Build history of the part. All positions in model axes, mm. Face numbers are marked on the shaded views. A direction names the side the tool comes from. Give positions to 0.01 mm unless a question says otherwise; leave off trailing zeros. Write each loop counter-clockwise with the first axis right and the second up, starting at its lowest first coordinate (ties: lowest second). Pieces come first, ordered by that corner, then holes. Notation, with made-up numbers: (88, 48.25) -> (125, 48.25) arc R17 cw to (125, 77.25) -> close; hole circle Ø4 at (84, 74). An arc over 180 degrees is marked (long way). Write item = value, one per line. Start each with the question number.
Q1. Tool access for the marked faces 1 and 2: list every direction of +Z, -Z, +X, -X, +Y, -Y with a clear straight run to the whole face (end or side of a thin tool).
Q2. Saw through at B-B, the plane z = 58. List the corners of the cut face in (x, y), then the cut area to 3 significant figures.
Q3. Saw through at D-D, the plane z = 139. List the corners of the cut face in (x, y).
Q4. Wall check: line 1 (Y direction, x = 21, z = -143); line 2 (X direction, y = 10.5, z = -98.5); line 3 (Y direction, x = -23, z = -87.5). Give the ranges that are in metal, low to high.
Q5. Drop flat-ended pins along their axis: P1, Ø6, axis at y = 5, z = 59.5, coming from the +X side; P2, Ø1.7, axis at y = 4.5, z = -142, coming from the -X side; P3, Ø12, axis at x = -7, z = -20, coming from the +Y side; P4, Ø6, axis at x = 12, z = -29.5, coming from the -Y side. Give the stop position or say it passes through.
Q6. Saw through at C-C, the plane z = -123. List the corners of the cut face in (x, y).
Q7. Saw through at A-A, the plane z = -68. List the corners of the cut face in (x, y), then the cut area to 3 significant figures.
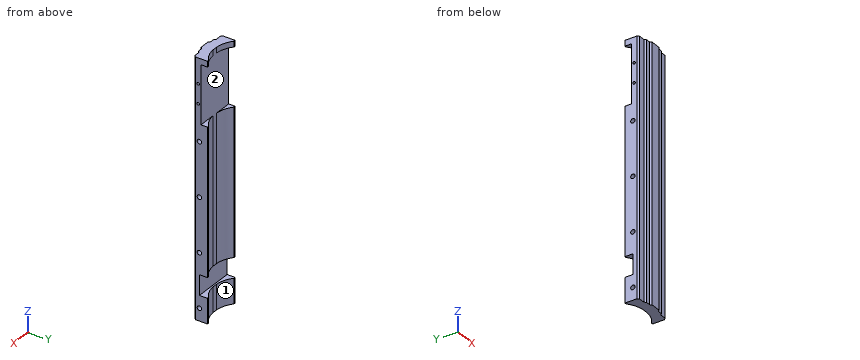
from build123d import *

# Parameters (mm, degrees)
SKETCH1_W               = 50
SKETCH1_H               = 317
BOSS_EXTRUDE1_DEPTH     = 7
BOSS_EXTRUDE2_DEPTH     = 317
SKETCH4_W               = 50
SKETCH4_H               = 72.5
CUT_EXTRUDE2_DEPTH      = 15
CUT_EXTRUDE3_DEPTH      = 12.5
CUT_EXTRUDE3_DEPTH_BACK = 2
SKETCH5_W               = 50
SKETCH5_H               = 25
SKETCH6_R               = 1.6
CUT_EXTRUDE4_DEPTH      = 4.5
SKETCH7_R               = 2.8
CUT_EXTRUDE5_DEPTH      = 9.1
LPATTERN2_COUNT         = 4
LPATTERN2_PITCH         = 67
MIRROR3_COPY_1_SKETCH_R = 2.8
MIRROR3_COPY_1_DEPTH    = 9.1
MIRROR3_COPY_2_SKETCH_R = 2.8
MIRROR3_COPY_2_DEPTH    = 9.1
MIRROR3_COPY_3_SKETCH_R = 2.8
MIRROR3_COPY_3_DEPTH    = 9.1
BOSS_EXTRUDE3_DEPTH     = 317


with BuildPart() as part:
    # Sketch1 → Boss-Extrude1 (new body)
    with BuildSketch(Plane(origin=(0, 0, 0), x_dir=(1, 0, 0), z_dir=(0, 1, 0))):
        Rectangle(SKETCH1_W, SKETCH1_H)
    extrude(amount=BOSS_EXTRUDE1_DEPTH)

    # Sketch2 → Boss-Extrude2 (add)
    with BuildSketch(Plane.XY.offset(158.5)):
        with BuildLine():
            Line((25, 0), (25, 15))
            Line((25, 15), (23, 15))
            ThreePointArc((23, 15), (12.243394569, 8.789970948), (-0.047456713, 7))
            Line((-0.047456713, 7), (-0.047456713, 0))
            Line((-0.047456713, 0), (25, 0))
        make_face()
    boss_extrude2 = extrude(amount=-BOSS_EXTRUDE2_DEPTH)

    # Mirror1: Boss-Extrude2 across plane
    add(boss_extrude2.mirror(Plane(origin=(0, 0, 0), x_dir=(0, 0, 1), z_dir=(1, 0, 0))))

    # Sketch4 → Cut-Extrude2 (cut)
    with BuildSketch(Plane(origin=(0, 7, 0), x_dir=(1, 0, 0), z_dir=(0, 1, 0))):
        with Locations((0, -115.25)):
            Rectangle(SKETCH4_W, SKETCH4_H)
    extrude(amount=CUT_EXTRUDE2_DEPTH, mode=Mode.SUBTRACT)

    # Sketch5 → Cut-Extrude3 (cut, two sides: drawn at the far end of the back side and taken through both)
    with BuildSketch(Plane(origin=(0, 7, 0), x_dir=(1, 0, 0), z_dir=(0, 1, 0)).offset(-CUT_EXTRUDE3_DEPTH_BACK)):
        with Locations((0, 115)):
            Rectangle(SKETCH5_W, SKETCH5_H)
    extrude(amount=CUT_EXTRUDE3_DEPTH + CUT_EXTRUDE3_DEPTH_BACK, mode=Mode.SUBTRACT)

    # Sketch6 → Cut-Extrude4 (cut)
    with BuildSketch(Plane.ZY.offset(25)):
        with Locations((103.166666667, 3.5)):
            Circle(SKETCH6_R)
        with Locations((127.333333333, 3.5)):
            Circle(SKETCH6_R)
    cut_extrude4 = extrude(amount=-CUT_EXTRUDE4_DEPTH, mode=Mode.SUBTRACT)

    # Sketch7 → Cut-Extrude5 (cut)
    with BuildSketch(Plane(origin=(25, 0, 0), x_dir=(0, 0, -1), z_dir=(1, 0, 0))):
        with Locations((143, 5)):
            Circle(SKETCH7_R)
    cut_extrude5 = extrude(amount=-CUT_EXTRUDE5_DEPTH, mode=Mode.SUBTRACT)

    # LPattern2: Cut-Extrude5 ×4
    with Locations(*[(0, 0, i * LPATTERN2_PITCH) for i in range(1, LPATTERN2_COUNT)]):
        add(cut_extrude5, mode=Mode.SUBTRACT)

    # Mirror3: Cut-Extrude4, Cut-Extrude5 across plane
    add(cut_extrude4.mirror(Plane(origin=(0, 0, 0), x_dir=(0, 0, 1), z_dir=(1, 0, 0))), mode=Mode.SUBTRACT)
    add(cut_extrude5.mirror(Plane(origin=(0, 0, 0), x_dir=(0, 0, 1), z_dir=(1, 0, 0))), mode=Mode.SUBTRACT)

    # Mirror3 copy 1 sketch → Mirror3 copy 1 (cut)
    with BuildSketch(Plane(origin=(-25, 0, 67), x_dir=(0, 0, -1), z_dir=(-1, 0, 0))):
        with Locations((143, -5)):
            Circle(MIRROR3_COPY_1_SKETCH_R)
    extrude(amount=-MIRROR3_COPY_1_DEPTH, mode=Mode.SUBTRACT)

    # Mirror3 copy 2 sketch → Mirror3 copy 2 (cut)
    with BuildSketch(Plane(origin=(-25, 0, 134), x_dir=(0, 0, -1), z_dir=(-1, 0, 0))):
        with Locations((143, -5)):
            Circle(MIRROR3_COPY_2_SKETCH_R)
    extrude(amount=-MIRROR3_COPY_2_DEPTH, mode=Mode.SUBTRACT)

    # Mirror3 copy 3 sketch → Mirror3 copy 3 (cut)
    with BuildSketch(Plane(origin=(-25, 0, 201), x_dir=(0, 0, -1), z_dir=(-1, 0, 0))):
        with Locations((143, -5)):
            Circle(MIRROR3_COPY_3_SKETCH_R)
    extrude(amount=-MIRROR3_COPY_3_DEPTH, mode=Mode.SUBTRACT)

    # Sketch8 → Boss-Extrude3 (add)
    with BuildSketch(Plane.XY.offset(158.5)):
        Polygon((23, -2), (15.5, -2), (13.5, -4), (8, -4), (6, -6), (0, -6), (0, 0), (25, 0), align=None)
    boss_extrude3 = extrude(amount=-BOSS_EXTRUDE3_DEPTH)

    # Mirror4: Boss-Extrude3 across plane
    add(boss_extrude3.mirror(Plane(origin=(0, 0, 0), x_dir=(0, 0, 1), z_dir=(1, 0, 0))))


solid = part.part
Report:
q1.face_1 = +Z, -Z, +Y
q1.face_2 = +Y
q2.outline = (-25, 0) -> (-23, -2) -> (-15.5, -2) -> (-13.5, -4) -> (-8, -4) -> (-6, -6) -> (6, -6) -> (8, -4) -> (13.5, -4) -> (15.5, -2) -> (23, -2) -> (25, 0) -> (25, 2.2) -> (15.9, 2.2) -> (15.9, 7.8) -> (25, 7.8) -> (25, 15) -> (23, 15) arc R32.97 cw to (2.91, 7) -> (-2.91, 7) arc R32.97 cw to (-23, 15) -> (-25, 15) -> (-25, 7.8) -> (-15.9, 7.8) -> (-15.9, 2.2) -> (-25, 2.2) -> close
q2.area = 570 mm2
q3.outline = (-25, 0) -> (-23, -2) -> (-15.5, -2) -> (-13.5, -4) -> (-8, -4) -> (-6, -6) -> (6, -6) -> (8, -4) -> (13.5, -4) -> (15.5, -2) -> (23, -2) -> (25, 0) -> (25, 7) -> (-25, 7) -> close
q4.line_1 = -2 to 2.2, 7.8 to 13.4
q4.line_2 = -25 to -16.28, 16.28 to 25
q4.line_3 = -2 to 15
q5.P1 = 25
q5.P2 = -15.9
q5.P3 = 9.06
q5.P4 = -4
q6.outline = (-25, 0) -> (-23, -2) -> (-15.5, -2) -> (-13.5, -4) -> (-8, -4) -> (-6, -6) -> (6, -6) -> (8, -4) -> (13.5, -4) -> (15.5, -2) -> (23, -2) -> (25, 0) -> (25, 5) -> (-25, 5) -> close
q7.outline = (-25, 0) -> (-23, -2) -> (-15.5, -2) -> (-13.5, -4) -> (-8, -4) -> (-6, -6) -> (6, -6) -> (8, -4) -> (13.5, -4) -> (15.5, -2) -> (23, -2) -> (25, 0) -> (25, 15) -> (23, 15) arc R32.97 cw to (2.91, 7) -> (-2.91, 7) arc R32.97 cw to (-23, 15) -> (-25, 15) -> close
q7.area = 672 mm2
